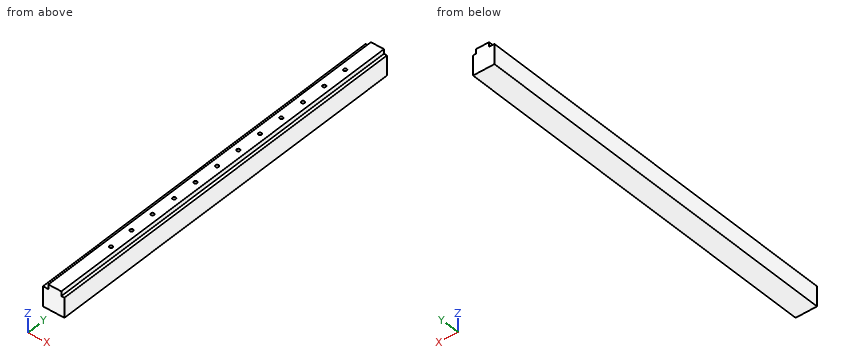
```python
from build123d import *

# Parameters (mm, degrees)
PAD010_DEPTH   = 500
SKETCH024_R    = 2.1
HOLE005_DEPTH  = 25
HOLE005_TIPS_R = 2.1


with BuildPart() as part:
    # Sketch023 → Pad010 (new body)
    with BuildSketch(Plane.XZ):
        Polygon((7, 0), (24, 0), (24, -6), (28, -6), (28, -32), (0, -32), (0, -6), (7, -6), align=None)
    extrude(amount=PAD010_DEPTH)

    # Sketch024 → Hole005 (cut)
    with BuildSketch(Plane.XY):
        with Locations((16.5, -414)):
            Circle(SKETCH024_R)
        with Locations((15.5, -381)):
            Circle(SKETCH024_R)
        with Locations((15, -348)):
            Circle(SKETCH024_R)
        with Locations((15.5, -315)):
            Circle(SKETCH024_R)
        with Locations((15.5, -282)):
            Circle(SKETCH024_R)
        with Locations((15.5, -248.5)):
            Circle(SKETCH024_R)
        with Locations((15.5, -215.5)):
            Circle(SKETCH024_R)
        with Locations((15.5, -182)):
            Circle(SKETCH024_R)
        with Locations((15.5, -149)):
            Circle(SKETCH024_R)
        with Locations((16, -116)):
            Circle(SKETCH024_R)
        with Locations((16, -83)):
            Circle(SKETCH024_R)
        with Locations((15.5, -50)):
            Circle(SKETCH024_R)
    extrude(amount=-HOLE005_DEPTH, mode=Mode.SUBTRACT)

    # Hole005 tips → Hole005 tip 1 section 0
    with BuildSketch(Plane.XY.offset(-25), mode=Mode.PRIVATE) as hole005_tip_1_s0:
        with Locations((16.5, -414)):
            Circle(HOLE005_TIPS_R)
    loft([hole005_tip_1_s0.sketch, Vertex(16.5, -414, -26.261807)], mode=Mode.SUBTRACT)

    # Hole005 tips → Hole005 tip 2 section 0
    with BuildSketch(Plane.XY.offset(-25), mode=Mode.PRIVATE) as hole005_tip_2_s0:
        with Locations((15.5, -381)):
            Circle(HOLE005_TIPS_R)
    loft([hole005_tip_2_s0.sketch, Vertex(15.5, -381, -26.261807)], mode=Mode.SUBTRACT)

    # Hole005 tips → Hole005 tip 3 section 0
    with BuildSketch(Plane.XY.offset(-25), mode=Mode.PRIVATE) as hole005_tip_3_s0:
        with Locations((15, -348)):
            Circle(HOLE005_TIPS_R)
    loft([hole005_tip_3_s0.sketch, Vertex(15, -348, -26.261807)], mode=Mode.SUBTRACT)

    # Hole005 tips → Hole005 tip 4 section 0
    with BuildSketch(Plane.XY.offset(-25), mode=Mode.PRIVATE) as hole005_tip_4_s0:
        with Locations((15.5, -315)):
            Circle(HOLE005_TIPS_R)
    loft([hole005_tip_4_s0.sketch, Vertex(15.5, -315, -26.261807)], mode=Mode.SUBTRACT)

    # Hole005 tips → Hole005 tip 5 section 0
    with BuildSketch(Plane.XY.offset(-25), mode=Mode.PRIVATE) as hole005_tip_5_s0:
        with Locations((15.5, -282)):
            Circle(HOLE005_TIPS_R)
    loft([hole005_tip_5_s0.sketch, Vertex(15.5, -282, -26.261807)], mode=Mode.SUBTRACT)

    # Hole005 tips → Hole005 tip 6 section 0
    with BuildSketch(Plane.XY.offset(-25), mode=Mode.PRIVATE) as hole005_tip_6_s0:
        with Locations((15.5, -248.5)):
            Circle(HOLE005_TIPS_R)
    loft([hole005_tip_6_s0.sketch, Vertex(15.5, -248.5, -26.261807)], mode=Mode.SUBTRACT)

    # Hole005 tips → Hole005 tip 7 section 0
    with BuildSketch(Plane.XY.offset(-25), mode=Mode.PRIVATE) as hole005_tip_7_s0:
        with Locations((15.5, -215.5)):
            Circle(HOLE005_TIPS_R)
    loft([hole005_tip_7_s0.sketch, Vertex(15.5, -215.5, -26.261807)], mode=Mode.SUBTRACT)

    # Hole005 tips → Hole005 tip 8 section 0
    with BuildSketch(Plane.XY.offset(-25), mode=Mode.PRIVATE) as hole005_tip_8_s0:
        with Locations((15.5, -182)):
            Circle(HOLE005_TIPS_R)
    loft([hole005_tip_8_s0.sketch, Vertex(15.5, -182, -26.261807)], mode=Mode.SUBTRACT)

    # Hole005 tips → Hole005 tip 9 section 0
    with BuildSketch(Plane.XY.offset(-25), mode=Mode.PRIVATE) as hole005_tip_9_s0:
        with Locations((15.5, -149)):
            Circle(HOLE005_TIPS_R)
    loft([hole005_tip_9_s0.sketch, Vertex(15.5, -149, -26.261807)], mode=Mode.SUBTRACT)

    # Hole005 tips → Hole005 tip 10 section 0
    with BuildSketch(Plane.XY.offset(-25), mode=Mode.PRIVATE) as hole005_tip_10_s0:
        with Locations((16, -116)):
            Circle(HOLE005_TIPS_R)
    loft([hole005_tip_10_s0.sketch, Vertex(16, -116, -26.261807)], mode=Mode.SUBTRACT)

    # Hole005 tips → Hole005 tip 11 section 0
    with BuildSketch(Plane.XY.offset(-25), mode=Mode.PRIVATE) as hole005_tip_11_s0:
        with Locations((16, -83)):
            Circle(HOLE005_TIPS_R)
    loft([hole005_tip_11_s0.sketch, Vertex(16, -83, -26.261807)], mode=Mode.SUBTRACT)

    # Hole005 tips → Hole005 tip 12 section 0
    with BuildSketch(Plane.XY.offset(-25), mode=Mode.PRIVATE) as hole005_tip_12_s0:
        with Locations((15.5, -50)):
            Circle(HOLE005_TIPS_R)
    loft([hole005_tip_12_s0.sketch, Vertex(15.5, -50, -26.261807)], mode=Mode.SUBTRACT)


with BuildPart() as part_1:
    # Body007 placement: moved
    add(part.part.moved(Location((309, 420, 35))))


solid = part_1.part
```
Could you check a few things on this model? Use its own coordinates, in mm. Coordinates: 2 decimals unless noted, no trailing zeros. Write each loop counter-clockwise with the first axis right and the second up, starting at its lowest first coordinate (ties: lowest second). Pieces come first, ordered by that corner, then holes. Notation, with made-up numbers: (0.25, 16) -> (38.25, 16) arc R31 ccw to (38.25, 46) -> close; hole circle Ø2 at (40, 75). An arc over 180 degrees is marked (long way). One line per question, with ' | ' between items. Start each with the question number.
1. Please list where these lines run through material, in increasing order: line 1 along X through (y, z) = (303.5, 11.5); line 2 along X through (y, z) = (39, 28); line 3 along Z through (x, y) = (334, 305).
2. Will these pins go through, and if not, where does the flat tip stop? P1, Ø3.5, axis at x = 325.5, y = 6, coming from the +Z side; P2, Ø2.5, axis at x = 324.5, y = 271, coming from the +Z side; P3, Ø3, axis at y = 66.5, z = 31.5, coming from the +X side.
3. If we section it at A-A (y = -34): Please give me the cut outline in (x, z).
Return value:
1) line 1: x = 309 to 322.96, 327.04 to 337 | line 2: x = 309 to 322.4, 326.6 to 337 | line 3: z = 3 to 29
2) P1: stops at z = 9.79 | P2: stops at z = 9.49 | P3: stops at x = 333
3) outline: (309, 3) -> (337, 3) -> (337, 29) -> (333, 29) -> (333, 35) -> (316, 35) -> (316, 29) -> (309, 29) -> close
